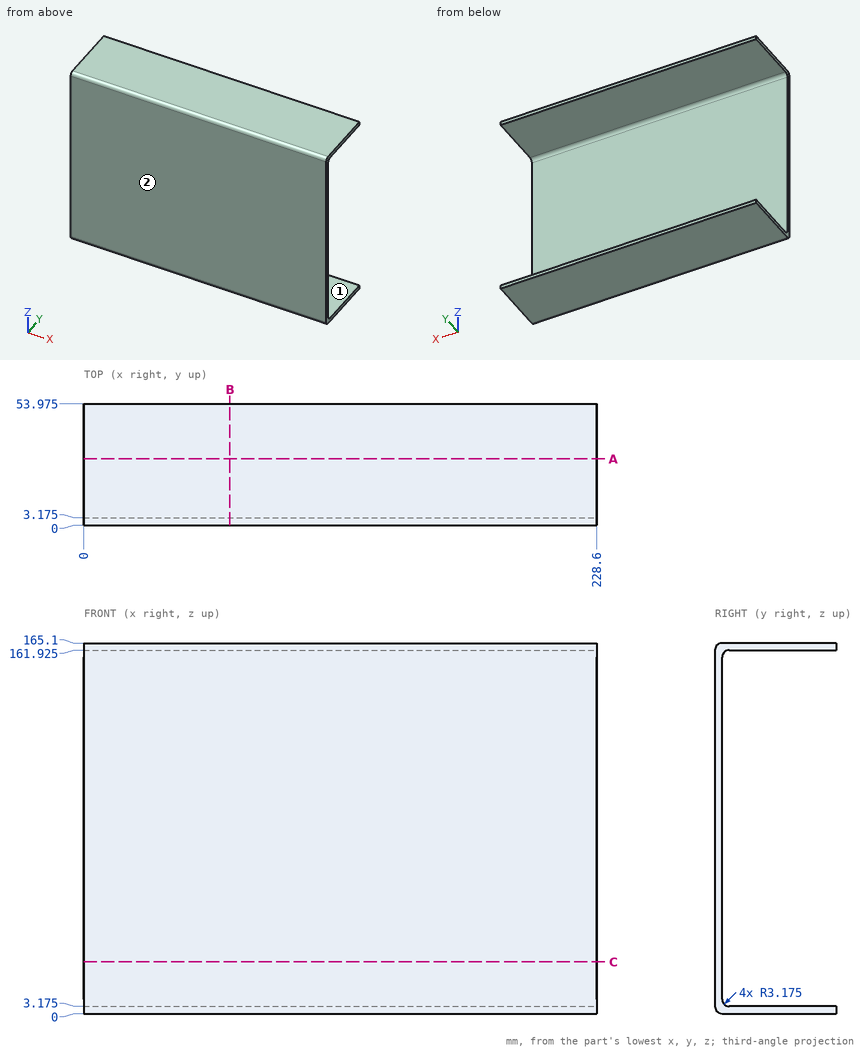
Design review of the part shown in the three views and the two pictorial views. Dimensions are in mm from the part's minimum x, y and z. A direction names the side the tool comes from. Give positions to 0.01 mm unless a question says otherwise; leave off trailing zeros. Loops run counter-clockwise (first coordinate to the right, second up) from the corner with the lowest first, then second, coordinate; pieces in that order, holes last. Notation, with made-up numbers: M 63.25,77.25 L 119.25,77.25 A25 ccw 119.25,109.25 Z; hole C 86.25,-9 d5. An arc over 180 degrees is marked long. Answer as a JSON object with one key per item and string values. Group by question number.
Q1. Insertion check: P1, Ø2, axis at x = 181, z = 111.5, coming from the +Y side (3 decimals). The pin has a flat end and moves straight along its axis. Give the tip position at first contact, or say it passes through.
Q2. Add section A-A on y = 29.5. Give the boundary of the cut face in (x, z) (3 decimals).
Q3. Add section C-C on z = 23. Give the boundary of the cut face in (x, y) (3 decimals).
Q4. Tool access review of the marked faces 1 and 2: name each direction out of +Z, -Z, +X, -X, +Y, -Y from which nothing blocks a thin tool from reaching the whole face with its end or side.
Q5. Add section B-B on x = 65. Give the boundary of the cut face in (y, z) (3 decimals), and give its area (3 significant figures).
Q6. For probe 1 along Z at (x, y) = (101, 42) (3 decimals); probe 2 along Y at (x, z) = (138.5, 136) (3 decimals), list the stretches that pass through material, from the lowest coordinate up. Write a range as [from, to].
Checked values:
{
 "1": {"P1": "y = 3.175"},
 "2": {"outline": "M 0,0 L 228.6,0 L 228.6,3.175 L 0,3.175 Z; M 0,161.925 L 228.6,161.925 L 228.6,165.1 L 0,165.1 Z"},
 "3": {"outline": "M 0,0 L 228.6,0 L 228.6,3.175 L 0,3.175 Z"},
 "4": {"face 1": "+X, -X, +Y", "face 2": "+Z, -Z, +X, -X, -Y"},
 "5": {"outline": "M 0,3.175 A3.175 ccw 3.175,0 L 53.975,0 L 53.975,3.175 L 6.35,3.175 A3.175 cw 3.175,6.35 L 3.175,158.75 A3.175 cw 6.35,161.925 L 53.975,161.925 L 53.975,165.1 L 3.175,165.1 A3.175 ccw 0,161.925 Z", "area": "847 mm²"},
 "6": {"probe 1": "[0, 3.175], [161.925, 165.1]", "probe 2": "[0, 3.175]"}
}
